Check sheet for the modelled part. Datum: model origin and axes. Units: mm. A direction names the side the tool comes from. Give positions to 0.01 mm unless a question says otherwise; leave off trailing zeros. Order: outer loops, then holes, each group sorted by start corner. A loop starts at its lowest first (then second) coordinate and runs counter-clockwise, first axis right, second up.
```python
from build123d import *

# Parameters (mm, degrees)
IZIM2_R               = 4
KES_EKSTR_ZYON2_DEPTH = 74.116345765


with BuildPart() as part:
    # Çizim1 → Döndür2 (revolve)
    with BuildSketch(Plane.XY, mode=Mode.PRIVATE) as d_nd_r2_sk:
        with BuildLine():
            Line((-1.500885478, 45), (1.970188902, 39))
            Line((1.970188902, 39), (5.970188902, 39))
            Line((5.970188902, 39), (8.499114522, 45))
            Line((8.499114522, 45), (11.499114522, 45))
            ThreePointArc((11.499114522, 45), (12.913328084, 44.414213562), (13.499114522, 43))
            Line((13.499114522, 43), (13.499114522, 27.5))
            Line((13.499114522, 27.5), (16.499114522, 27.5))
            ThreePointArc((16.499114522, 27.5), (17.913328084, 26.914213562), (18.499114522, 25.5))
            Line((18.499114522, 25.5), (18.499114522, 20.020661157))
            Line((18.499114522, 20.020661157), (18.499114522, 7.5))
            Line((18.499114522, 7.5), (-22.500885478, 7.5))
            Line((-22.500885478, 7.5), (-22.500885478, 15.5))
            ThreePointArc((-22.500885478, 15.5), (-21.915099041, 16.914213562), (-20.500885478, 17.5))
            Line((-20.500885478, 17.5), (-6.500885478, 17.5))
            Line((-6.500885478, 17.5), (-6.500885478, 24.44214876))
            Line((-6.500885478, 24.44214876), (-6.500885478, 43))
            ThreePointArc((-6.500885478, 43), (-5.915099041, 44.414213562), (-4.500885478, 45))
            Line((-4.500885478, 45), (-1.500885478, 45))
        make_face()
    revolve(d_nd_r2_sk.sketch.rotate(Axis((-33.856257379, 0, 0), (1, 0, 0)), 90), axis=Axis((-33.856257379, 0, 0), (1, 0, 0)))

    # Çizim2 → Kes-Ekstrüzyon2 (cut, through all)
    with BuildSketch(Plane(origin=(13.499114522, 0, 0), x_dir=(0, 0, -1), z_dir=(1, 0, 0))):
        with Locations((0, 34.402169776)):
            Circle(IZIM2_R)
        with Locations((29.793152971, -17.201084888)):
            Circle(IZIM2_R)
        with Locations((-29.793152971, -17.201084888)):
            Circle(IZIM2_R)
    extrude(amount=-KES_EKSTR_ZYON2_DEPTH, mode=Mode.SUBTRACT)


solid = part.part
```
(1) Tool access check on faces 1 (the face through (-6.501, -1, -19)), 2 (the face through (1.8, 34.86, 18.13)), 3 (the face through (3.639, 37.775, -2.15)), 4 (the face through (13.499, -1, 28)). Record the directions out of +Z, -Z, +X, -X, +Y, -Y that give a thin tool (end or side, any length) a straight path to the whole face; none if there is none.
(2) Go/stop test with flat-tipped pins: P1, Ø4, axis at x = -12, y = 9, coming from the -Z side; P2, Ø10.5, axis at y = 34.4, z = 0, coming from the -X side; P3, Ø1, axis at x = -16, y = 4, coming from the +Z side; P4, Ø5, axis at y = -17.2, z = 29.79, coming from the +X side. Record where each tip stops, or that it passes through.
(3) Release check for a two-part mould opening along Y. For faces 5 (the face through (18.499, -6, 5)), 6 (the face through (3.998, -38.668, -5.077)), 7 (the face through (3.64, -17.03, 33.79)) record: released by +Y, released by -Y, zero draft, split by the parting line, or undercut.
(4) Thickness scan on L1, parallel to Y at x = 5, z = 0; L2, parallel to Y at x = 4, z = 1; L3, parallel to Z at x = -5.5, y = -15.5. Record the ranges inside material, lowest first.
(5) Sectioned sample at C-C (z = 0). Count the separate pieces of the cut face and the enclosed holes in it, plus the area to 3 significant figures.
(6) Sectioned sample at B-B (x = -9). Enter the section's corners in (y, z).
Values follow:
1. face 1: -X
1. face 2: none
1. face 3: +X, -X
1. face 4: +X
2. P1: stops at z = -16.04
2. P2: stops at x = -6.5
2. P3: stops at z = 17.15
2. P4: passes through
3. face 5: zero draft
3. face 6: split by the parting line
3. face 7: undercut
4. L1: y = -39 to -7.5, 7.5 to 30.4, 38.4 to 39
4. L2: y = -38.99 to -7.43, 7.43 to 30.53, 38.28 to 38.99
4. L3: z = -41.96 to -33.41, -26.17 to 26.17, 33.41 to 41.96
5. separate pieces: 3
5. enclosed holes: 0
5. area: 1,770 mm2
6. outline: circle Ø35 at (0, 0); hole circle Ø15 at (0, 0)
